Geometry check sheet. Reference: the model listing, model coordinates, mm. Coordinates: 2 decimals unless noted, no trailing zeros. Write each loop counter-clockwise with the first axis right and the second up, starting at its lowest first coordinate (ties: lowest second). Pieces come first, ordered by that corner, then holes.
from build123d import *

# Parameters (mm, degrees)
F0_W     = 177.8
F0_H     = 88.9
F1_DEPTH = 50.8
F2_R     = 25.4
F3_DEPTH = 25.4
F4_R     = 19.05
F5_DEPTH = 25.4


with BuildPart() as f1:
    # F0 (on Top) → F1 (new body)
    with BuildSketch(Plane.XY):
        with Locations((88.9, 44.45)):
            Rectangle(F0_W, F0_H)
    extrude(amount=F1_DEPTH)

    # F2 (on face) → F3 (join)
    with BuildSketch(Plane.XY.offset(50.8)):
        with Locations((44.45, 44.45)):
            Circle(F2_R)
    extrude(amount=F3_DEPTH)

    # F4 (on face) → F5 (cut)
    with BuildSketch(Plane.XY.offset(50.8)):
        with Locations((127, 38.1)):
            Circle(F4_R)
    extrude(amount=-F5_DEPTH, mode=Mode.SUBTRACT)


solid = f1.part
1. Sectioned sample at B-B, the plane z = 43.5. Record the boundary of the cut face in (x, y).
Computed values:
outline: (0, 0) - (177.8, 0) - (177.8, 88.9) - (0, 88.9) - close; hole circle Ø38.1 at (127, 38.1)
2. Sectioned sample at C-C, the plane y = 41. Record the boundary of the cut face in (x, z).
Computed values:
outline: (0, 0) - (177.8, 0) - (177.8, 50.8) - (145.83, 50.8) - (145.83, 25.4) - (108.17, 25.4) - (108.17, 50.8) - (69.61, 50.8) - (69.61, 76.2) - (19.29, 76.2) - (19.29, 50.8) - (0, 50.8) - close
3. Sectioned sample at A-A, the plane x = 44.45. Record the boundary of the cut face in (y, z).
Computed values:
outline: (0, 0) - (88.9, 0) - (88.9, 50.8) - (69.85, 50.8) - (69.85, 76.2) - (19.05, 76.2) - (19.05, 50.8) - (0, 50.8) - close
4. Gauge pin test, flat ends, axial feed: pin 1 Ø12 at (y, z) = (46, 61) entering from -X; pin 2 Ø10 at (x, y) = (109, 43) entering from +Z; pin 3 Ø11.5 at (x, y) = (127, 32) entering from +Z. Record the tip position at first contact, or that the pin passes through.
Computed values:
pin 1: stops at x = 19.05
pin 2: stops at z = 50.8
pin 3: stops at z = 25.4
5. Draft check along Y on faces 1 (the cylindrical face through (135.79, 21.2, 38.28)), 2 (the flat face through (127, 38, 25.4)), 3 (the cylindrical face through (38.944, 19.654, 63.322)), 4 (the flat face through (88, 45, 0)). Enter one of: released by +Y, released by -Y, zero draft, split by the parting line, or undercut.
Computed values:
face 1: undercut
face 2: undercut
face 3: split by the parting line
face 4: zero draft
6. Sectioned sample at D-D, the plane z = 70. Record the boundary of the cut face in (x, y).
Computed values:
outline: circle Ø50.8 at (44.45, 44.45)
7. Thickness scan on line 1 along X through (y, z) = (38, 41); line 2 along Y through (x, z) = (127, 34); line 3 along Z through (x, y) = (104.5, 44). Record the ranges inside material, lowest first.
Computed values:
line 1: x = 0 to 107.95, 146.05 to 177.8
line 2: y = 0 to 19.05, 57.15 to 88.9
line 3: z = 0 to 50.8
